Design review of the part shown in the three views and the two pictorial views. Dimensions are in mm from the part's minimum x, y and z. Coordinates: 2 decimals unless noted, no trailing zeros. Order: outer loops, then holes, each group sorted by start corner. A loop starts at its lowest first (then second) coordinate and runs counter-clockwise, first axis right, second up. Notation, with made-up numbers: (28, 65) - (49, 65) arc R18 cw to (49, 77) - close; hole circle Ø9 at (83.25, 63). An arc over 180 degrees is marked (long way). One line per item, written item: value. Start each with the question number.
(1) Clearance check with flat-ended pins moving along their axes: pin 1 (2 mm diameter, centred on y = 40, z = 3, fed in from +X); pin 2 (3 mm diameter, centred on x = 47.5, z = 1, fed in from -Y); pin 3 (2 mm diameter, centred on x = 32, z = 4, fed in from +Y); pin 4 (1 mm diameter, centred on x = 19.5, z = 1.5, fed in from +Y). State where each tip first meets the part, or that it passes through.
(2) Consider section A-A on x = 40. Write out the cut boundary in (y, z).
(3) To check wall thickness, follow line 1 along X through (y, z) = (21.5, 2.75); line 2 along X through (y, z) = (48.5, 3); line 3 along Y through (x, z) = (4, 3). State the ranges of each line that lie inside material, in increasing order.
(4) Mouldability with a two-part tool opening along X and no side actions: class the marked faces 1, 2 and 3 as released by +X, released by -X, zero draft, split by the parting line, or undercut.
(5) Consider section D-D on x = 64.5. Write out the cut boundary in (y, z).
(6) Consider section C-C on y = 9.5. Write out the cut boundary in (x, z), then the cut area to 3 significant figures.
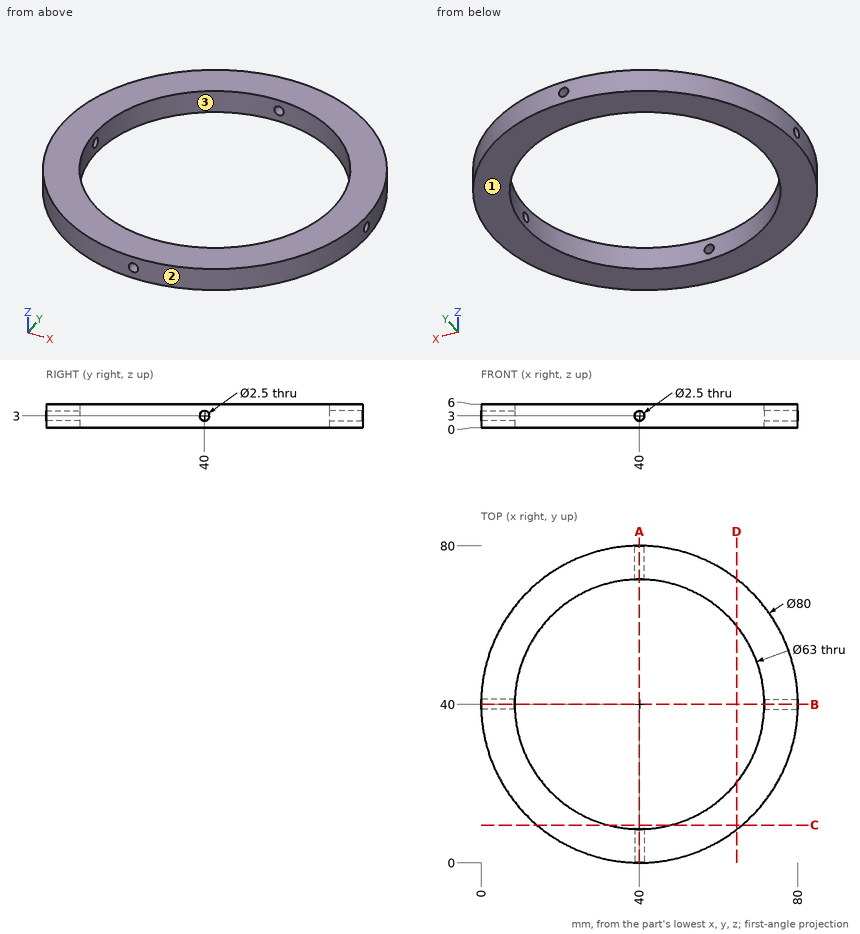
Geometry check:
1. pin 1: passes through
1. pin 2: stops at y = 0.45
1. pin 3: stops at y = 79.38
1. pin 4: stops at y = 74.64
2. outline: (0, 0) - (8.5, 0) - (8.5, 1.75) - (0, 1.75) - close; (0, 4.25) - (8.5, 4.25) - (8.5, 6) - (0, 6) - close; (71.5, 0) - (80, 0) - (80, 1.75) - (71.5, 1.75) - close; (71.5, 4.25) - (80, 4.25) - (80, 6) - (71.5, 6) - close
3. line 1: x = 4.54 to 14.5, 65.5 to 75.46
3. line 2: x = 0.91 to 9.67, 70.33 to 79.09
3. line 3: y = 22.56 to 38.75, 41.25 to 57.44
4. face 1: zero draft
4. face 2: split by the parting line
4. face 3: undercut
5. outline: (8.38, 0) - (20.2, 0) - (20.2, 6) - (8.38, 6) - close; (59.8, 0) - (71.62, 0) - (71.62, 6) - (59.8, 6) - close
6. outline: (14.12, 0) - (32.13, 0) - (32.13, 6) - (14.12, 6) - close; (47.87, 0) - (65.88, 0) - (65.88, 6) - (47.87, 6) - close
6. area: 216 mm^2
